from build123d import *

# Parameters (mm, degrees)
BOSS_EXTRUDE1_DEPTH = 1


with BuildPart() as part:
    # Sketch1 → Boss-Extrude1 (new body)
    with BuildSketch(Plane.XY):
        with BuildLine():
            Line((0, 0), (23, 0))
            Line((23, 0), (23, 215))
            ThreePointArc((23, 215), (21.535533906, 218.535533906), (18, 220))
            Line((18, 220), (5, 220))
            ThreePointArc((5, 220), (1.464466094, 218.535533906), (0, 215))
            Line((0, 215), (0, 202.619429464))
            ThreePointArc((0, 202.619429464), (0.554995555, 200.329902115), (2.096774194, 198.548645766))
            ThreePointArc((2.096774194, 198.548645766), (6.495941299, 190.291918226), (2.5625, 181.803440127))
            ThreePointArc((2.5625, 181.803440127), (2.147918272, 181.282022055), (2, 180.632503002))
            Line((2, 180.632503002), (2, 179.367496998))
            ThreePointArc((2, 179.367496998), (2.147918272, 178.717977945), (2.5625, 178.196559873))
            ThreePointArc((2.5625, 178.196559873), (6.5, 170), (2.5625, 161.803440127))
            ThreePointArc((2.5625, 161.803440127), (2.147918272, 161.282022055), (2, 160.632503002))
            Line((2, 160.632503002), (2, 159.367496998))
            ThreePointArc((2, 159.367496998), (2.147918272, 158.717977945), (2.5625, 158.196559873))
            ThreePointArc((2.5625, 158.196559873), (6.5, 150), (2.5625, 141.803440127))
            ThreePointArc((2.5625, 141.803440127), (2.147918272, 141.282022055), (2, 140.632503002))
            Line((2, 140.632503002), (2, 139.367496998))
            ThreePointArc((2, 139.367496998), (2.147918272, 138.717977945), (2.5625, 138.196559873))
            ThreePointArc((2.5625, 138.196559873), (6.5, 130), (2.5625, 121.803440127))
            ThreePointArc((2.5625, 121.803440127), (2.147918272, 121.282022055), (2, 120.632503002))
            Line((2, 120.632503002), (2, 119.367496998))
            ThreePointArc((2, 119.367496998), (2.147918272, 118.717977945), (2.5625, 118.196559873))
            ThreePointArc((2.5625, 118.196559873), (6.5, 110), (2.5625, 101.803440127))
            ThreePointArc((2.5625, 101.803440127), (2.147918272, 101.282022055), (2, 100.632503002))
            Line((2, 100.632503002), (2, 99.367496998))
            ThreePointArc((2, 99.367496998), (2.147918272, 98.717977945), (2.5625, 98.196559873))
            ThreePointArc((2.5625, 98.196559873), (6.5, 90), (2.5625, 81.803440127))
            ThreePointArc((2.5625, 81.803440127), (2.147918272, 81.282022055), (2, 80.632503002))
            Line((2, 80.632503002), (2, 79.367496998))
            ThreePointArc((2, 79.367496998), (2.147918272, 78.717977945), (2.5625, 78.196559873))
            ThreePointArc((2.5625, 78.196559873), (6.5, 70), (2.5625, 61.803440127))
            ThreePointArc((2.5625, 61.803440127), (2.147918272, 61.282022055), (2, 60.632503002))
            Line((2, 60.632503002), (2, 59.367496998))
            ThreePointArc((2, 59.367496998), (2.147918272, 58.717977945), (2.5625, 58.196559873))
            ThreePointArc((2.5625, 58.196559873), (6.495941299, 49.708081774), (2.096774194, 41.451354234))
            ThreePointArc((2.096774194, 41.451354234), (0.554995555, 39.670097885), (0, 37.380570536))
            Line((0, 37.380570536), (0, 0))
        make_face()
    extrude(amount=BOSS_EXTRUDE1_DEPTH)


solid = part.part
The listing builds one solid part. Answer for the finished solid, in the listing's coordinates (mm). Round coordinates to 2 decimals unless told otherwise and drop trailing zeros. Order: outer loops, then holes, each group sorted by start corner. A loop starts at its lowest first (then second) coordinate and runs counter-clockwise, first axis right, second up. Notation, with made-up numbers: (0, 51.25) -> (53, 51.25) arc R26 cw to (53, 74.25) -> close; hole circle Ø10 at (76, 87). An arc over 180 degrees is marked (long way). One line per item, written item: value.
Item 1: Find section A-A, the plane y = 186. Give the vertices of the cut face in (x, z).
Taken from the geometry:
outline: (5.71, 0) -> (23, 0) -> (23, 1) -> (5.71, 1) -> close
Item 2: Find section B-B, the plane y = 107.5. Give the vertices of the cut face in (x, z).
Taken from the geometry:
outline: (6.2, 0) -> (23, 0) -> (23, 1) -> (6.2, 1) -> close
Item 3: For a pull along Y with two mould halves and no side action, classify faces 1 (the cylindrical face through (1.5, 218.57, 0.49)), 2 (the cylindrical face through (6.5, 150.1, 0.5)), 3 (the cylindrical face through (6.5, 130.1, 0.5)), 4 (the flat face through (14, 112, 1)) as released by +Y, released by -Y, zero draft, split by the parting line, or undercut.
Taken from the geometry:
face 1: released by +Y
face 2: undercut
face 3: undercut
face 4: zero draft
Item 4: Given P1, Ø8, axis at x = 19.5, y = 126, coming from the -Z side; P2, Ø0.5, axis at y = 80, z = 0.5, coming from the -X side, each flat-ended and moving along its own axis, determine where each tip first touches the part or whether it passes through.
Taken from the geometry:
P1: stops at z = 0
P2: stops at x = 2
Item 5: Straight lines are drawn through the part: L1, parallel to X at y = 50, z = 0.15; L2, parallel to X at y = 75, z = 0.4; L3, parallel to Y at x = 19.75, z = 0.55. For each, find the intervals that lie inside material, in ascending order.
Taken from the geometry:
L1: x = 6.5 to 23
L2: x = 5.23 to 23
L3: y = 0 to 219.68
